Design review of the part built by this model. Coordinates are the model's own, in mm. Round coordinates to 2 decimals unless told otherwise and drop trailing zeros. Order: outer loops, then holes, each group sorted by start corner. A loop starts at its lowest first (then second) coordinate and runs counter-clockwise, first axis right, second up. Notation, with made-up numbers: (-28.75, 35.5) - (22.25, 35.5) arc R23 ccw to (22.25, 50.5) - close; hole circle Ø11 at (66, -9). An arc over 180 degrees is marked (long way). Write item = value, one per line.
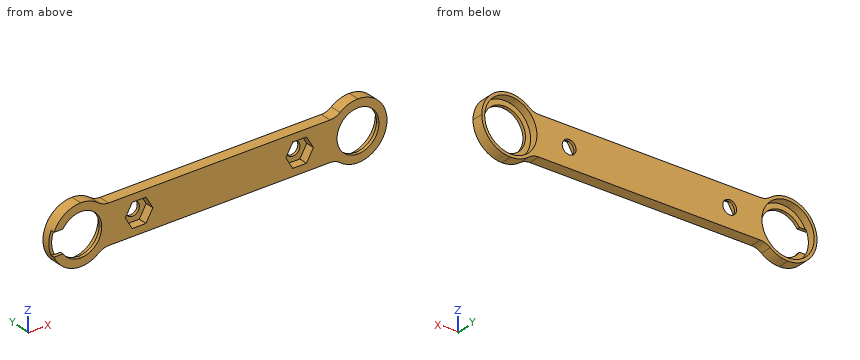
from build123d import *

# Parameters (mm, degrees)
F1_DEPTH = 3.55
F2_R     = 8.1
F3_DEPTH = 2.55
F4_R     = 5
F5_R     = 2.15
F6_DEPTH = 2.7
F7_DEPTH = 3.551
F8_W     = 1.2
F8_H     = 7
F9_DEPTH = 200


# Not quite as in the source:
# - a feature names something its author has since deleted; it is built from what else it names


with BuildPart() as f1:
    # F0 (on Front) → F1 (new body)
    with BuildSketch(Plane.XZ):
        with BuildLine():
            Line((0, 6.5), (0, 9))
            ThreePointArc((0, 9), (-9, 0), (0, -9))
            Line((0, -9), (0, -6.5))
            ThreePointArc((0, -6.5), (-6.5, 0), (0, 6.5))
        make_face()
        with BuildLine():
            ThreePointArc((6.7082039325, -6), (8.4075512307, -3.211398808), (9, 0))
            ThreePointArc((9, 0), (8.4075512307, 3.211398808), (6.7082039325, 6))
            ThreePointArc((6.7082039325, 6), (3.6742346142, 8.2158383626), (0, 9))
            Line((0, 9), (0, 6.5))
            ThreePointArc((0, 6.5), (4.5961940777, 4.5961940777), (6.5, 0))
            ThreePointArc((6.5, 0), (4.5961940777, -4.5961940777), (0, -6.5))
            Line((0, -6.5), (0, -9))
            ThreePointArc((0, -9), (3.6742346142, -8.2158383626), (6.7082039325, -6))
        make_face()
        with BuildLine():
            ThreePointArc((86, 9), (82.3257653858, 8.2158383626), (79.2917960675, 6))
            ThreePointArc((79.2917960675, 6), (77, 0), (79.2917960675, -6))
            ThreePointArc((79.2917960675, -6), (82.3257653858, -8.2158383626), (86, -9))
            Line((86, -9), (86, -6.5))
            ThreePointArc((86, -6.5), (79.5, 0), (86, 6.5))
            Line((86, 6.5), (86, 9))
        make_face()
        with BuildLine():
            ThreePointArc((95, 0), (92.3639610307, 6.3639610307), (86, 9))
            Line((86, 9), (86, 6.5))
            ThreePointArc((86, 6.5), (90.5961940777, 4.5961940777), (92.5, 0))
            ThreePointArc((92.5, 0), (90.5961940777, -4.5961940777), (86, -6.5))
            Line((86, -6.5), (86, -9))
            ThreePointArc((86, -9), (92.3639610307, -6.3639610307), (95, 0))
        make_face()
        with BuildLine():
            ThreePointArc((6.7082039325, 6), (8.4075512307, 3.211398808), (9, 0))
            ThreePointArc((9, 0), (8.4075512307, -3.211398808), (6.7082039325, -6))
            Line((6.7082039325, -6), (79.2917960675, -6))
            ThreePointArc((79.2917960675, -6), (77, 0), (79.2917960675, 6))
            Line((79.2917960675, 6), (6.7082039325, 6))
        make_face()
    extrude(amount=F1_DEPTH)

    # F2 (on face) → F3 (cut)
    with BuildSketch(Plane.XZ):
        Circle(F2_R)
        with Locations((86, 0)):
            Circle(F2_R)
    extrude(amount=F3_DEPTH, mode=Mode.SUBTRACT)

    # F4
    f4_edges = [f1.edges().sort_by_distance(p)[0] for p in [
        (6.708204, -1.775, -6),
        (6.708204, -1.775, 6),
        (79.291796, -1.775, 6),
        (79.291796, -1.775, -6),
    ]]
    fillet(f4_edges, radius=F4_R)

    # F5 (on face) → F6 (cut)
    with BuildSketch(Plane.XZ.offset(3.55)):
        Polygon((22.372391992, 0), (20.236195996, 3.7), (15.963804004, 3.7), (13.827608008, 0), (15.963804004, -3.7), (20.236195996, -3.7), align=None)
        with Locations((18.1, 0)):
            Circle(F5_R, mode=Mode.SUBTRACT)
        Polygon((63.627608008, 0), (65.763804004, -3.7), (70.036195996, -3.7), (72.172391992, 0), (70.036195996, 3.7), (65.763804004, 3.7), align=None)
        with Locations((67.9, 0)):
            Circle(F5_R, mode=Mode.SUBTRACT)
    extrude(amount=-F6_DEPTH, mode=Mode.SUBTRACT)

    # F5 (on face) → F7 (cut, through all)
    with BuildSketch(Plane.XZ.offset(3.55)):
        with Locations((18.1, 0)):
            Circle(F5_R)
        with Locations((67.9, 0)):
            Circle(F5_R)
    extrude(amount=-F7_DEPTH, mode=Mode.SUBTRACT)

    # F8 (on Right) → F9 (cut)
    with BuildSketch(Plane.YZ):
        with Locations((-2.95, 0)):
            Rectangle(F8_W, F8_H)
    extrude(amount=-F9_DEPTH, mode=Mode.SUBTRACT)


solid = f1.part
Item 1: For line 1 along X through (y, z) = (-0.65, 1.5); line 2 along Z through (x, y) = (86, -0.9); line 3 along X through (y, z) = (-2.65, 4.5), list the stretches that pass through material, from the lowest coordinate up. Write a range as [from, to].
Data:
line_1 = [-8.87, -7.96], [7.96, 16.56], [19.64, 66.36], [69.44, 78.04], [93.96, 94.87]
line_2 = [-9, -8.1], [8.1, 9]
line_3 = [-7.79, -4.69], [4.69, 81.31], [90.69, 93.79]
Item 2: Take a section at C-C, the plane z = 5. State the section outline as (x, y) points, and give its area (3 significant figures).
Data:
outline = (-7.48, -3.55) - (-4.15, -3.55) - (-4.15, -2.55) - (-6.37, -2.55) - (-6.37, 0) - (-7.48, 0) - close; (4.15, -3.55) - (81.85, -3.55) - (81.85, -2.55) - (79.63, -2.55) - (79.63, 0) - (6.37, 0) - (6.37, -2.55) - (4.15, -2.55) - close; (90.15, -3.55) - (93.48, -3.55) - (93.48, 0) - (92.37, 0) - (92.37, -2.55) - (90.15, -2.55) - close
area = 277 mm2
Item 3: Take a section at A-A, the plane x = 67.9. State the section outline as (y, z) points.
Data:
outline = (-3.55, -6) - (0, -6) - (0, -2.15) - (-0.85, -2.15) - (-0.85, -3.7) - (-3.55, -3.7) - close; (-3.55, 3.7) - (-0.85, 3.7) - (-0.85, 2.15) - (0, 2.15) - (0, 6) - (-3.55, 6) - close
Item 4: Take a section at B-B, the plane y = -1.7. State the section outline as (x, z) points, and give its area (3 significant figures).
Data:
outline = (5.57, -7.07) arc R5 cw to (8.66, -6) - (77.34, -6) arc R5 cw to (80.43, -7.07) arc R9 ccw (long way) to (80.43, 7.07) arc R5 cw to (77.34, 6) - (8.66, 6) arc R5 cw to (5.57, 7.07) arc R9 ccw (long way) to start; hole circle Ø16.2 at (0, 0); hole (13.83, 0) - (15.96, -3.7) - (20.24, -3.7) - (22.37, 0) - (20.24, 3.7) - (15.96, 3.7) - close; hole (63.63, 0) - (65.76, -3.7) - (70.04, -3.7) - (72.17, 0) - (70.04, 3.7) - (65.76, 3.7) - close; hole circle Ø16.2 at (86, 0)
area = 837 mm2
Item 5: Take a section at D-D, the plane x = 12.5. State the section outline as (y, z) points.
Data:
outline = (-3.55, -6) - (0, -6) - (0, 6) - (-3.55, 6) - close
Item 6: Insertion check: P1, Ø2, axis at x = 17, y = -2, coming from the -Z side; P2, Ø2, axis at x = 18.5, y = -2, coming from the +Z side; P3, Ø1.3, axis at x = -6.5, y = -3, coming from the -Z side. Each pin has a flat end and moves straight along its axis. Give the tip position at first contact, or say it passes through.
Data:
P1 = -6
P2 = 6
P3 = -6.84
